Verification items for the finished model (mm, model axes). Face numbers are marked on the shaded views. A direction names the side the tool comes from. Round coordinates to 2 decimals unless told otherwise and drop trailing zeros. Loops run counter-clockwise (first coordinate to the right, second up) from the corner with the lowest first, then second, coordinate; pieces in that order, holes last. Notation, with made-up numbers: M 14.5,24.5 L 42.5,24.5 A19 cw 42.5,42.5 Z; hole C 31.25,28.25 d3. An arc over 180 degrees is marked long. Write item = value, one per line. Start each with the question number.
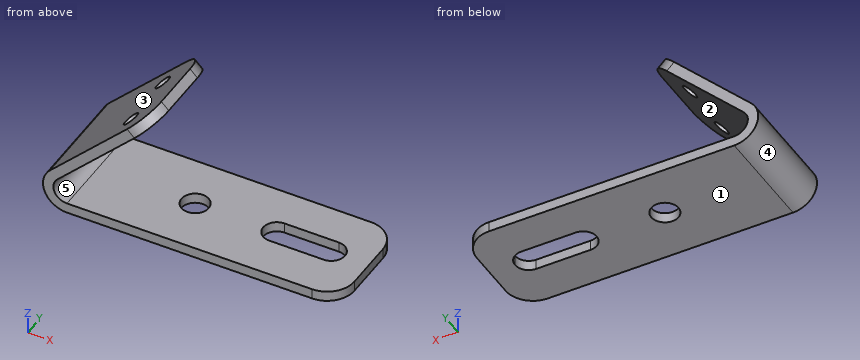
from build123d import *

# Parameters (mm, degrees)
F1_DEPTH = 19.5
F2_R     = 2.5
F3_DEPTH = 25
F4_R     = 1.5
F5_DEPTH = 12
F6_R     = 5


with BuildPart() as f1:
    # F0 (on Front) → F1 (new body)
    with BuildSketch(Plane.XZ):
        with BuildLine():
            Line((-50, 0), (0, 0))
            Line((0, 0), (0, 1.9))
            Line((0, 1.9), (-50, 1.9))
            ThreePointArc((-50, 1.9), (-52.309699, 3.443291), (-51.767767, 6.167767))
            Line((-51.767767, 6.167767), (-34.090097, 23.845436))
            Line((-34.090097, 23.845436), (-35.4336, 25.188939))
            Line((-35.4336, 25.188939), (-53.11127, 7.51127))
            ThreePointArc((-53.11127, 7.51127), (-54.06507, 2.716193), (-50, 0))
        make_face()
    extrude(amount=F1_DEPTH)

    # F2 (on face) → F3 (cut)
    with BuildSketch(Plane.XY.offset(1.9)):
        with BuildLine():
            ThreePointArc((-17, -12.025), (-15.232233, -11.292767), (-14.5, -9.525))
            ThreePointArc((-14.5, -9.525), (-15.232233, -7.757233), (-17, -7.025))
            ThreePointArc((-17, -7.025), (-19.5, -9.525), (-17, -12.025))
        make_face()
        with BuildLine():
            ThreePointArc((-17, -7.025), (-15.232233, -7.757233), (-14.5, -9.525))
            ThreePointArc((-14.5, -9.525), (-15.232233, -11.292767), (-17, -12.025))
            Line((-17, -12.025), (-7, -12.025))
            ThreePointArc((-7, -12.025), (-9.5, -9.525), (-7, -7.025))
            Line((-7, -7.025), (-17, -7.025))
        make_face()
        with BuildLine():
            ThreePointArc((-4.5, -9.525), (-5.232233, -7.757233), (-7, -7.025))
            ThreePointArc((-7, -7.025), (-9.5, -9.525), (-7, -12.025))
            ThreePointArc((-7, -12.025), (-5.232233, -11.292767), (-4.5, -9.525))
        make_face()
        with Locations((-32, -9.525)):
            Circle(F2_R)
    extrude(amount=-F3_DEPTH, mode=Mode.SUBTRACT)

    # F4 (on face) → F5 (cut)
    with BuildSketch(Plane(origin=(-30.31127, 0, 30.31127), x_dir=(0, -1, 0), z_dir=(-0.707107, 0, 0.707107))):
        with Locations((4.5, -14.744069)):
            Circle(F4_R)
        with Locations((15, -14.744069)):
            Circle(F4_R)
    extrude(amount=-F5_DEPTH, mode=Mode.SUBTRACT)

    # F6
    f6_edges = [f1.edges().sort_by_distance(p)[0] for p in [
        (-34.761849, 0, 24.517188),
        (-34.761849, -19.5, 24.517188),
        (0, -19.5, 0.95),
        (0, 0, 0.95),
    ]]
    fillet(f6_edges, radius=F6_R)


solid = f1.part
1. Mould release check, pull along Z, two halves, no side actions. Record for the marked faces 3, 4 and 5: pulls with the +Z half, pulls with the -Z half, needs draft (parallel to the pull), parting line crosses it, or undercut.
2. Thickness scan on line 1 (X direction, y = -7.5, z = 1.75); line 2 (Y direction, x = -32, z = 1.4) (3 decimals); line 3 (Z direction, x = -27, y = -7.5). Record the ranges inside material, lowest first.
3. Section check C-C, the plane x = -40. Give the number of separate pieces and of enclosed holes in the cut face, and give its area (3 significant figures).
4. Tool access check on the marked faces 1 and 2. Record the directions out of +Z, -Z, +X, -X, +Y, -Y that give a thin tool (end or side, any length) a straight path to the whole face; none if there is none.
5. Gauge pin test, flat ends, axial feed: P1, Ø2, axis at y = -10, z = 13, coming from the +X side; P2, Ø3, axis at y = -12.5, z = 15, coming from the +X side; P3, Ø3, axis at y = -10.5, z = 9.5, coming from the +X side. Record the tip position at first contact, or that the pin passes through.
6. Section check B-B, the plane y = -15.25. Enter the section's corners in (x, z), and give its area (3 significant figures).
7. Section check D-D, the plane z = 13.5. Enter the section's corners in (x, y), and give its area (3 significant figures).
8. Section check A-A, the plane x = -32. Enter the section's corners in (y, z) (3 decimals).
Computed values:
q1.face_3 = pulls with the +Z half
q1.face_4 = parting line crosses it
q1.face_5 = undercut
q2.line_1 = -53.51 to -33.47, -30.53 to -18.47, -5.53 to 0
q2.line_2 = -19.5 to -12.025, -7.025 to 0
q2.line_3 = 0 to 1.9
q3.separate_pieces = 4
q3.enclosed_holes = 0
q3.area = 74.5 mm2
q4.face_1 = -Z, +X, -X, +Y, -Y
q4.face_2 = +X, +Y, -Y
q5.P1 = -43.94
q5.P2 = -41.44
q5.P3 = -46.94
q6.outline = M -53.11,7.51 A4.4 ccw -50,0 L -0.06,0 L -0.06,1.9 L -50,1.9 A2.5 cw -51.77,6.17 L -40.44,17.5 L -41.78,18.84 Z; M -39.69,20.93 L -38.35,19.59 L -34.13,23.81 L -35.47,25.15 Z
q6.area = 152 mm2
q7.outline = M -47.12,-19.5 L -44.44,-19.5 L -44.44,0 L -47.12,0 Z
q7.area = 52.4 mm2
q8.outline = M -19.5,0 L -12.025,0 L -12.025,1.9 L -19.5,1.9 Z; M -7.025,0 L 0,0 L 0,1.9 L -7.025,1.9 Z
